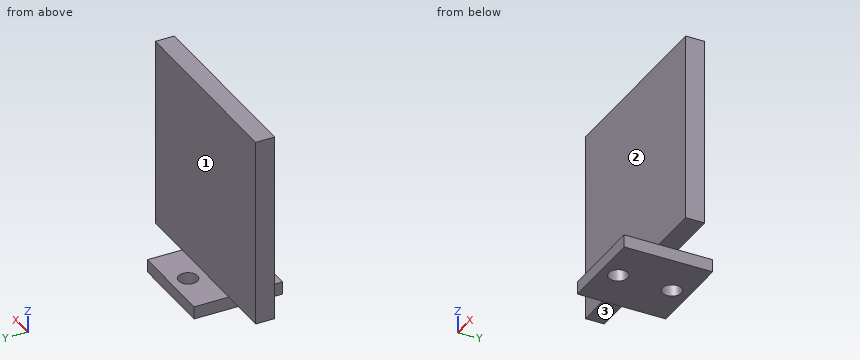
from build123d import *

# Parameters (mm, degrees)
SKETCH1_W             = 14
SKETCH1_H             = 14
BOSS_EXTRUDE1_DEPTH   = 2
SKETCH2_W             = 30
SKETCH2_H             = 3
BOSS_EXTRUDE2_DEPTH   = 30
F_3_0MM_DOWEL_HOLE1_D = 3


with BuildPart() as part:
    # Sketch1 → Boss-Extrude1 (new body)
    with BuildSketch(Plane.XY):
        Rectangle(SKETCH1_W, SKETCH1_H)
    extrude(amount=BOSS_EXTRUDE1_DEPTH)

    # Sketch2 → Boss-Extrude2 (add)
    with BuildSketch(Plane.XY.offset(2)):
        Rectangle(SKETCH2_W, SKETCH2_H)
    extrude(amount=BOSS_EXTRUDE2_DEPTH)

    # Ø3.0mm Dowel Hole1 (through all)
    with Locations(Plane.XY.offset(2)):
        with Locations((0, -4.25), (0, 4.25)):
            Hole(F_3_0MM_DOWEL_HOLE1_D / 2)


solid = part.part
Read the model definition and answer for the solid it produces. Units are mm, in the model's axes. Face numbers are marked on the shaded views. A direction names the side the tool comes from. Coordinates: 2 decimals unless noted, no trailing zeros. Loops run counter-clockwise (first coordinate to the right, second up) from the corner with the lowest first, then second, coordinate; pieces in that order, holes last. Notation, with made-up numbers: (-16, 70) -> (4, 70) arc R12 cw to (4, 89) -> close; hole circle Ø3 at (30.5, 35). An arc over 180 degrees is marked (long way). Answer in a Markdown table with one row per item.
Item 1: A cutting plane is placed at C-C on x = -6. Determine the outline of the cut face in (y, z).
Returned:
| item | result |
|---|---|
| outline | (-7, 0) -> (7, 0) -> (7, 2) -> (1.5, 2) -> (1.5, 32) -> (-1.5, 32) -> (-1.5, 2) -> (-7, 2) -> close |
Item 2: A cutting plane is placed at A-A on y = 4.25. Determine the outline of the cut face in (x, z).
Returned:
| item | result |
|---|---|
| outline | (-7, 0) -> (-1.5, 0) -> (-1.5, 2) -> (-7, 2) -> close; (1.5, 0) -> (7, 0) -> (7, 2) -> (1.5, 2) -> close |
Item 3: A cutting plane is placed at D-D on z = 16. Determine the outline of the cut face in (x, y), plus the area to 3 significant figures.
Returned:
| item | result |
|---|---|
| outline | (-15, -1.5) -> (15, -1.5) -> (15, 1.5) -> (-15, 1.5) -> close |
| area | 90.0 mm^2 |
Item 4: For the marked faces 1, 2 and 3, determine the directions among +Z, -Z, +X, -X, +Y, -Y from which every point of the face is accessible in a straight line to the end or side of a thin tool.
Returned:
| item | result |
|---|---|
| face 1 | +Z, +X, -X, +Y |
| face 2 | +Z, +X, -X, -Y |
| face 3 | -Z, -X, +Y, -Y |
Item 5: Each of these flat-tipped pins is pushed along its axis until it touches: P1, Ø1.6, axis at y = 3, z = 1.5, coming from the +X side; P2, Ø0.6, axis at y = 1.5, z = 0.5, coming from the -X side; P3, Ø1.5, axis at x = -10.5, y = 0, coming from the -Z side; P4, Ø1.8, axis at x = 0, y = 4.25, coming from the +Z side. Where does it stop, or does it pass through?
Returned:
| item | result |
|---|---|
| P1 | stops at x = 7 |
| P2 | stops at x = -7 |
| P3 | stops at z = 2 |
| P4 | passes through |
Item 6: Straight lines are drawn through the part: line 1 along Y through (x, z) = (0, 0.7); line 2 along Z through (x, y) = (-8, 1.25); line 3 along Z through (x, y) = (5.75, -6.5). For each, find the intervals that lie inside material, in ascending order. Write a range as [from, to].
Returned:
| item | result |
|---|---|
| line 1 | y = [-7, -5.75], [-2.75, 2.75], [5.75, 7] |
| line 2 | z = [2, 32] |
| line 3 | z = [0, 2] |
Item 7: A cutting plane is placed at B-B on x = 0. Determine the outline of the cut face in (y, z), plus the area to 3 significant figures.
Returned:
| item | result |
|---|---|
| outline | (-7, 0) -> (-5.75, 0) -> (-5.75, 2) -> (-7, 2) -> close; (-2.75, 0) -> (2.75, 0) -> (2.75, 2) -> (1.5, 2) -> (1.5, 32) -> (-1.5, 32) -> (-1.5, 2) -> (-2.75, 2) -> close; (5.75, 0) -> (7, 0) -> (7, 2) -> (5.75, 2) -> close |
| area | 106 mm^2 |
